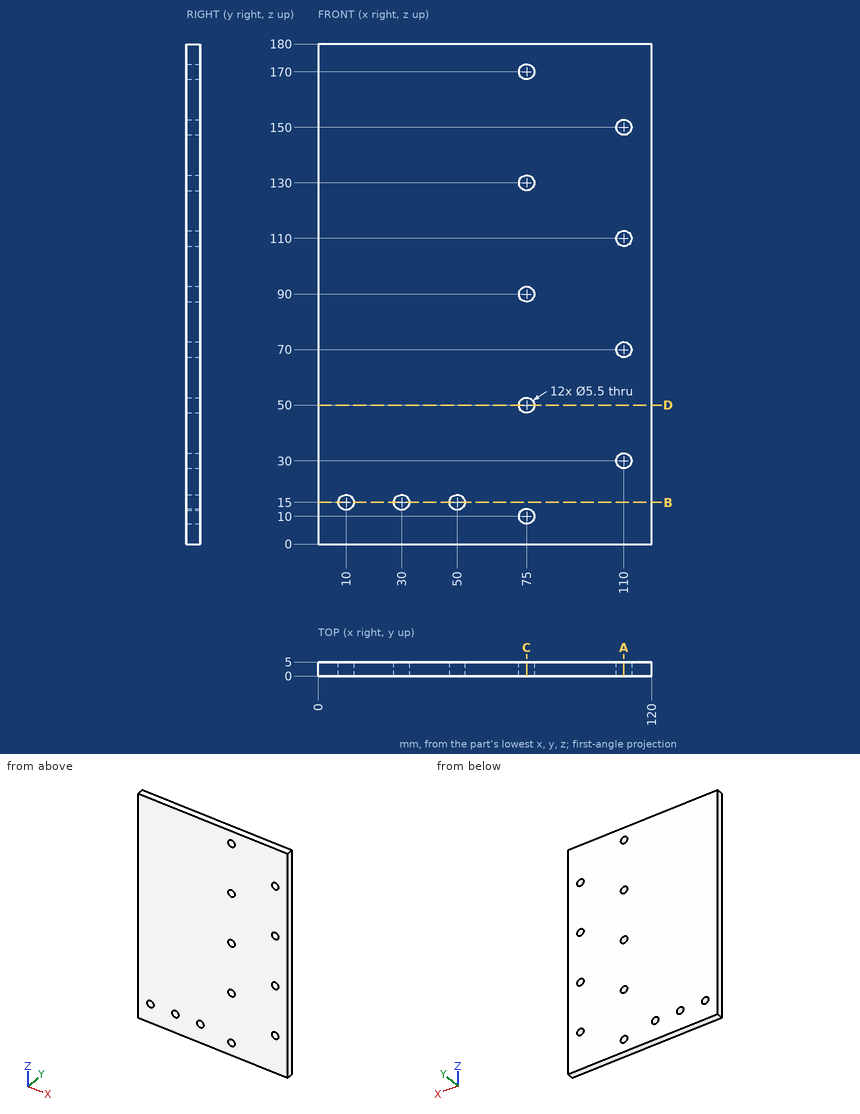
Could you check a few things on this drawing? It's one solid part, dimensions in mm from its lowest x, y, z. Give positions to 0.01 mm unless a question says otherwise; leave off trailing zeros. Order: outer loops, then holes, each group sorted by start corner. A loop starts at its lowest first (then second) coordinate and runs counter-clockwise, first axis right, second up. Notation, with made-up numbers: M 77.5,26 L 103.5,26 A20 cw 103.5,63 Z; hole C 70.5,21.25 d1. An arc over 180 degrees is marked long. Use one line per item in the form item = value. Start each with the question number.
Item 1: If I drill on line 1 along X through (y, z) = (1.25, 15); line 2 along Z through (x, y) = (75, 1.9); line 3 along Z through (x, y) = (110, 3.1), over which ranges is the centre line in solid material (lowest first)?
Item 2: Will this pin go through, and if not, where does the flat tip stop? pin 1 Ø3.5 at (x, z) = (10, 15) entering from +Y.
Item 3: If we section it at C-C (x = 75): Write out the boundary of the cut face in (y, z).
Item 4: If we section it at D-D (z = 50): Write out the boundary of the cut face in (x, y), then the cut area to 4 significant figures.
Item 5: If we section it at A-A (x = 110): Write out the boundary of the cut face in (y, z).
Item 6: If we section it at B-B (z = 15): Write out the boundary of the cut face in (x, y), then the cut area to 4 significant figures.
Outcome:
q1.line_1 = 0 to 7.25, 12.75 to 27.25, 32.75 to 47.25, 52.75 to 120
q1.line_2 = 0 to 7.25, 12.75 to 47.25, 52.75 to 87.25, 92.75 to 127.25, 132.75 to 167.25, 172.75 to 180
q1.line_3 = 0 to 27.25, 32.75 to 67.25, 72.75 to 107.25, 112.75 to 147.25, 152.75 to 180
q2.pin_1 = through
q3.outline = M 0,0 L 5,0 L 5,7.25 L 0,7.25 Z; M 0,12.75 L 5,12.75 L 5,47.25 L 0,47.25 Z; M 0,52.75 L 5,52.75 L 5,87.25 L 0,87.25 Z; M 0,92.75 L 5,92.75 L 5,127.25 L 0,127.25 Z; M 0,132.75 L 5,132.75 L 5,167.25 L 0,167.25 Z; M 0,172.75 L 5,172.75 L 5,180 L 0,180 Z
q4.outline = M 0,0 L 72.25,0 L 72.25,5 L 0,5 Z; M 77.75,0 L 120,0 L 120,5 L 77.75,5 Z
q4.area = 572.5 mm2
q5.outline = M 0,0 L 5,0 L 5,27.25 L 0,27.25 Z; M 0,32.75 L 5,32.75 L 5,67.25 L 0,67.25 Z; M 0,72.75 L 5,72.75 L 5,107.25 L 0,107.25 Z; M 0,112.75 L 5,112.75 L 5,147.25 L 0,147.25 Z; M 0,152.75 L 5,152.75 L 5,180 L 0,180 Z
q6.outline = M 0,0 L 7.25,0 L 7.25,5 L 0,5 Z; M 12.75,0 L 27.25,0 L 27.25,5 L 12.75,5 Z; M 32.75,0 L 47.25,0 L 47.25,5 L 32.75,5 Z; M 52.75,0 L 120,0 L 120,5 L 52.75,5 Z
q6.area = 517.5 mm2
